Autodesk Inventor part; units mm, degrees
ref_plane "YZ Plane" through (0, 0, 0) normal (1, 0, 0) x (0, 1, 0)
ref_plane "XZ Plane" through (0, 0, 0) normal (0, 1, 0) x (-1, 0, 0)
ref_plane "XY Plane" through (0, 0, 0) normal (0, 0, 1) x (1, 0, 0)
sketch "Sketch1" plane through (0, 0, 0) normal (0, 0, 1) x (1, 0, 0)
  line L0 (0, 0) -> (0, 20)
  line L1 (0, 20) -> (20, 20)
  line L2 (20, 20) -> (20, 60)
  line L3 (20, 60) -> (420, 60)
  line L4 (420, 60) -> (420, 20)
  line L5 (420, 20) -> (440, 20)
  line L6 (440, 20) -> (440, 0)
  line L7 (440, 0) -> (0, 0)
  dimension "d0" = 20
  dimension "d1" = 20
  dimension "d2" = 40
  dimension "d3" = 400
  dimension "d4" = 40
  dimension "d5" = 20
extrude "Extrusion1" add sketch "Sketch1" along normal blind 10
sketch "Sketch2" plane through (0, 0, 10) normal (0, 0, 1) x (1, 0, 0)
  line L0 (20, 60) -> (20, 20)
  line L1 (0, 0) -> (440, 0)
  point P0 (80, 10)
  dimension "d8" = 60
  dimension "d16" = 10
hole "Hole1" at (80, 10, 10) direction (0, 0, -1) diameter 10 end through all
sketch "Sketch3" plane through (0, 0, 10) normal (0, 0, 1) x (1, 0, 0)
  line L0 (420, 20) -> (420, 60)
  line L1 (0, 0) -> (440, 0)
  point P0 (360, 10)
  dimension "d17" = 60
  dimension "d25" = 10
hole "Hole2" at (360, 10, 10) direction (0, 0, -1) diameter 10 end through all
sketch "Sketch4" plane through (0, 0, 10) normal (0, 0, 1) x (1, 0, 0)
  line L0 (20, 60) -> (20, 20)
  line L1 (0, 0) -> (440, 0)
  point P0 (220, 30)
  dimension "d26" = 200
  dimension "d34" = 30
hole "Hole3" at (220, 30, 10) direction (0, 0, -1) diameter 20 end through all
Design review of the part built by this model. Coordinates are the model's own, in mm. A direction names the side the tool comes from. Round coordinates to 2 decimals unless told otherwise and drop trailing zeros. Write each loop counter-clockwise with the first axis right and the second up, starting at its lowest first coordinate (ties: lowest second). Pieces come first, ordered by that corner, then holes. Notation, with made-up numbers: (49, -12.5) -> (79, -12.5) arc R17 ccw to (79, -3.5) -> close; hole circle Ø3 at (22, 78.5). An arc over 180 degrees is marked (long way). Answer in a Markdown table with one row per item.
Q1. Take a section at D-D, the plane x = 220. State the section outline as (y, z) points.
The answers:
| item | result |
|---|---|
| outline | (0, 0) -> (20, 0) -> (20, 10) -> (0, 10) -> close; (40, 0) -> (60, 0) -> (60, 10) -> (40, 10) -> close |
Q2. To check wall thickness, follow L1, parallel to X at y = 10, z = 6.25; L2, parallel to Y at x = 220, z = 7.75; L3, parallel to X at y = 14.5, z = 4. State the ranges of each line that lie inside material, in increasing order. Write a range as [from, to].
The answers:
| item | result |
|---|---|
| L1 | [0, 75], [85, 355], [365, 440] |
| L2 | [0, 20], [40, 60] |
| L3 | [0, 77.82], [82.18, 357.82], [362.18, 440] |
Q3. Take a section at B-B, the plane y = 10. State the section outline as (x, z) points.
The answers:
| item | result |
|---|---|
| outline | (0, 0) -> (75, 0) -> (75, 10) -> (0, 10) -> close; (85, 0) -> (355, 0) -> (355, 10) -> (85, 10) -> close; (365, 0) -> (440, 0) -> (440, 10) -> (365, 10) -> close |
Q4. For faces 4 (the face through (430, 20, 5)), 5 (the face through (229.76, 32.17, 4.93)), 6 (the face through (10, 20, 5)), list the 3-axis set-ups (+Z, -Z, +X, -X, +Y, -Y) from which the entire face can be reached by the end or side of a thin tool; tool diameter is ignored.
The answers:
| item | result |
|---|---|
| face 4 | +Z, -Z, +X, +Y |
| face 5 | +Z, -Z |
| face 6 | +Z, -Z, -X, +Y |
Q5. Clearance check with flat-ended pins moving along their axes: pin 1 Ø3 at (y, z) = (52.5, 2.5) entering from +X; pin 2 Ø3 at (y, z) = (36.5, 1) entering from -X. State where each tip first meets the part, or that it passes through.
The answers:
| item | result |
|---|---|
| pin 1 | x = 420 |
| pin 2 | x = 20 |
Q6. Take a section at C-C, the plane z = 7.75. State the section outline as (x, y) points.
The answers:
| item | result |
|---|---|
| outline | (0, 0) -> (440, 0) -> (440, 20) -> (420, 20) -> (420, 60) -> (20, 60) -> (20, 20) -> (0, 20) -> close; hole circle Ø10 at (80, 10); hole circle Ø20 at (220, 30); hole circle Ø10 at (360, 10) |
Q7. Take a section at A-A, the plane x = 360. State the section outline as (y, z) points, then the cut area to 3 significant figures.
The answers:
| item | result |
|---|---|
| outline | (0, 0) -> (5, 0) -> (5, 10) -> (0, 10) -> close; (15, 0) -> (60, 0) -> (60, 10) -> (15, 10) -> close |
| area | 500 mm² |
Q8. Draft analysis for pull direction Y (two halves, no side actions). For faces 1 (the face through (84.88, 11.08, 4.93)), 2 (the face through (217, 60, 5)), 3 (the face through (420, 40, 5)), state which applies: +Y half, -Y half, draft (parallel to the pull), parting line (faces both ways), or undercut.
The answers:
| item | result |
|---|---|
| face 1 | undercut |
| face 2 | +Y half |
| face 3 | draft |
